CAD build for the part. Positions are in the model's coordinates, mm. A direction names the side the tool comes from. Coordinates: 2 decimals unless noted, no trailing zeros. Loops run counter-clockwise (first coordinate to the right, second up) from the corner with the lowest first, then second, coordinate; pieces in that order, holes last. Notation, with made-up numbers: (-23, -15.75) -> (12, -15.75) arc R11 cw to (12, -10.75) -> close; hole circle Ø4 at (-36.75, 0.5). An arc over 180 degrees is marked (long way). Answer as a JSON object with one key per item and string values. Group by question number.
from build123d import *

# Parameters (mm, degrees)
F0_W      = 12
F0_H      = 38.1
F1_DEPTH  = 50.8
F2_R      = 3.33175
F3_DEPTH  = 25.4
F4_W      = 25.4
F4_H      = 76.2
F4_W_2    = 38.1
F4_H_2    = 50.8
F4_W_3    = 12
F4_H_3    = 38.1
F4_H_4    = 25.4
F5_DEPTH  = 6.35
F7_DEPTH  = 1.905
F8_R      = 3.33175
F9_DEPTH  = 12.7
F10_R     = 5.08
F11_DEPTH = 15.24
F13_DEPTH = 2.54
F14_W     = 27.02
F14_H     = 33.02
F15_DEPTH = 6.351
F16_R     = 2.413
F17_DEPTH = 6.351


# Not quite as in the source:
# - a pattern or mirror of a feature is missing from the dataset's text; its kind, count and spacing are read off the source's solid


with BuildPart() as f1:
    # F0 (on Top) → F1 (new body)
    with BuildSketch(Plane.XY):
        Rectangle(F0_W, F0_H)
    extrude(amount=F1_DEPTH)

    # F2 (on face) → F3 (cut)
    with BuildSketch(Plane.XY.offset(50.8)):
        with Locations((0, 12.7)):
            Circle(F2_R)
        with Locations((0, -12.7)):
            Circle(F2_R)
    extrude(amount=-F3_DEPTH, mode=Mode.SUBTRACT)

    # F4 (on face) → F5 (join)
    with BuildSketch(Plane(origin=(0, 0, 0), x_dir=(1, 0, 0), z_dir=(0, 0, -1))):
        with Locations((0, 63.5)):
            Rectangle(F4_W, F4_H)
        with Locations((31.75, 0)):
            Rectangle(F4_W_2, F4_H_2)
        Rectangle(F4_W, F4_H_2)
        Rectangle(F4_W_3, F4_H_3, mode=Mode.SUBTRACT)
        with Locations((-31.75, 0)):
            Rectangle(F4_W_2, F4_H_2)
        with Locations((0, -38.1)):
            Rectangle(F4_W, F4_H_4)
    extrude(amount=-F5_DEPTH)

    # F6 (on Right) → F7 (join, symmetric)
    with BuildSketch(Plane.YZ):
        with BuildLine():
            Line((-19.05, 6.35), (-19.05, 22.86))
            add(Edge.make_bspline(
                [(-90.6148681487, 15.7624194539), (-19.05, 4.6606890297), (-19.05, 22.86)],
                knots=[4.0563179373, 4.0563179373, 4.0563179373, 6.2831853072, 6.2831853072, 6.2831853072], degree=2, weights=[1, 0.4415833544, 1]))
            ThreePointArc((-90.6148681487, 15.7624194539), (-98.2724942161, 13.5830277507), (-101.6, 6.35))
            Line((-101.6, 6.35), (-25.4, 6.35))
            Line((-25.4, 6.35), (-19.05, 6.35))
        make_face()
        with BuildLine():
            Line((19.05, 22.86), (19.05, 6.35))
            Line((19.05, 6.35), (25.4, 6.35))
            Line((25.4, 6.35), (50.8, 6.35))
            ThreePointArc((50.8, 6.35), (46.5346393393, 14.2911472106), (37.5586731715, 15.1200934946))
            add(Edge.make_bspline(
                [(19.05, 22.86), (19.05, 7.2770438497), (37.5586731715, 15.1200934946)],
                knots=[0, 0, 0, 2.0982208016, 2.0982208016, 2.0982208016], degree=2, weights=[1, 0.4983425099, 1]))
        make_face()
    extrude(amount=F7_DEPTH, both=True)

    # F8 (on face) → F9 (cut)
    with BuildSketch(Plane.XZ.offset(101.6)):
        with Locations((-7.62, 6.35)):
            Circle(F8_R)
        with Locations((7.62, 6.35)):
            Circle(F8_R)
    extrude(amount=-F9_DEPTH, mode=Mode.SUBTRACT)

    # F10 (on face) → F11 (join)
    with BuildSketch(Plane.XZ.offset(101.6)):
        with Locations((-7.62, 6.35)):
            Circle(F10_R)
        with BuildLine():
            ThreePointArc((-4.28825, 6.35), (-7.62, 3.01825), (-10.95175, 6.35))
            ThreePointArc((-10.95175, 6.35), (-7.62, 9.68175), (-4.28825, 6.35))
        make_face(mode=Mode.SUBTRACT)
        with Locations((7.62, 6.35)):
            Circle(F10_R)
        with BuildLine():
            ThreePointArc((10.95175, 6.35), (7.62, 3.01825), (4.28825, 6.35))
            ThreePointArc((4.28825, 6.35), (7.62, 9.68175), (10.95175, 6.35))
        make_face(mode=Mode.SUBTRACT)
    extrude(amount=-F11_DEPTH)

    # F12 (on face) → F13 (join)
    with BuildSketch(Plane(origin=(0, -86.36, 0), x_dir=(-1, 0, 0), z_dir=(0, 1, 0))):
        with BuildLine():
            ThreePointArc((-4.28825, 6.35), (-7.62, 9.68175), (-10.95175, 6.35))
            Line((-10.95175, 6.35), (-4.28825, 6.35))
        make_face()
        with BuildLine():
            ThreePointArc((10.95175, 6.35), (7.62, 9.68175), (4.28825, 6.35))
            Line((4.28825, 6.35), (10.95175, 6.35))
        make_face()
    extrude(amount=-F13_DEPTH)

    # F14 (on face) → F15 (cut, through all)
    with BuildSketch(Plane.XY.offset(6.35)):
        with Locations((-27.13, 0)):
            Rectangle(F14_W, F14_H)
        with Locations((28.4, 0)):
            Rectangle(F14_W, F14_H)
    extrude(amount=-F15_DEPTH, mode=Mode.SUBTRACT)

    # F16 (on face) → F17 (cut, through all)
    with BuildSketch(Plane.XY.offset(6.35)):
        with Locations((-7.3025, -73.66)):
            Circle(F16_R)
        with Locations((-7.3025, -38.1)):
            Circle(F16_R)
        with Locations((-45.72, -20.955)):
            Circle(F16_R)
        with Locations((-45.72, 20.955)):
            Circle(F16_R)
        with Locations((-7.3025, 38.1)):
            Circle(F16_R)
    f17 = extrude(amount=-F17_DEPTH, mode=Mode.SUBTRACT)

    # F17_copies: F17 across plane
    add(f17.mirror(Plane(origin=(0, 0, 0), x_dir=(0, 0, 1), z_dir=(1, 0, 0))), mode=Mode.SUBTRACT)


solid = f1.part
Item 1: Pull direction Z, two halves, no side cores. Call faces 1 (the cylindrical face through (-0.03, -98.18, 13.66)), 2 (the cylindrical face through (8.342, -95.339, 9.603)), 3 (the flat face through (-27, -16.51, 3)): +Z half, -Z half, draft (parallel to the pull), parting line (faces both ways), or undercut.
Item 2: Drill centre lines: L1, parallel to Y at x = 0, z = 46.5; L2, parallel to X at y = -38, z = 2; L3, parallel to X at y = -73, z = 3. Where is each one in solid material? Low to high.
Item 3: Band-saw the part on A-A, the plane x = 45.72. List the corners of the cut face in (y, z).
Item 4: 3-axis set-ups, long thin cutter, end or side, ignore diameter. For faces 4 (the flat face through (-32, 25.4, 3)), 5 (the flat face through (0, 19.05, 28)), 6 (the flat face through (1.905, 35, 11)), 7 (the flat face through (12.7, 38, 3)): which of +Z, -Z, +X, -X, +Y, -Y reach the whole face in a straight line?
Item 5: Band-saw the part on B-B, the plane y = -12.7. List the corners of the cut face in (x, z), and give its area (3 significant figures).
Item 6: Flat gauge pins, fed straight in: P1, Ø2.5, axis at x = -9.5, z = 9.5, coming from the +Y side; P2, Ø7.5, axis at x = 7.3, y = -38.1, coming from the +Z side; P3, Ø3, axis at x = -30, z = 2, coming from the +Y side; P4, Ø10.5, axis at x = 7.62, z = 6.35, coming from the -Y side. Where does each tip first touch, or does it go through?
Item 7: Band-saw the part on C-C, the plane x = -22. List the corners of the cut face in (y, z).
Item 8: Band-saw the part on D-D, the plane z = 29. List the corners of the cut face in (x, y), and give its area (3 significant figures).
Reply:
{
 "1": {"face 1": "+Z half", "face 2": "undercut", "face 3": "draft"},
 "2": {"L1": "-19.05 to -16.03, -9.37 to 9.37, 16.03 to 19.05", "L2": "-12.7 to -9.71, -4.89 to 4.89, 9.71 to 12.7", "L3": "-12.7 to -9.62, -4.98 to 4.98, 9.62 to 12.7"},
 "3": {"outline": "(-25.4, 0) -> (-23.37, 0) -> (-23.37, 6.35) -> (-25.4, 6.35) -> close; (-18.54, 0) -> (18.54, 0) -> (18.54, 6.35) -> (-18.54, 6.35) -> close; (23.37, 0) -> (25.4, 0) -> (25.4, 6.35) -> (23.37, 6.35) -> close"},
 "4": {"face 4": "+Z, -Z, -X, +Y", "face 5": "+Z, +Y", "face 6": "+Z, +X, +Y", "face 7": "+Z, -Z, +X, +Y"},
 "5": {"outline": "(-50.8, 0) -> (-40.64, 0) -> (-40.64, 6.35) -> (-50.8, 6.35) -> close; (-13.62, 0) -> (14.89, 0) -> (14.89, 6.35) -> (6, 6.35) -> (6, 50.8) -> (3.33, 50.8) -> (3.33, 25.4) -> (-3.33, 25.4) -> (-3.33, 50.8) -> (-6, 50.8) -> (-6, 6.35) -> (-13.62, 6.35) -> close; (41.91, 0) -> (50.8, 0) -> (50.8, 6.35) -> (41.91, 6.35) -> close", "area": "666 mm²"},
 "6": {"P1": "y = -86.36", "P2": "z = 6.35", "P3": "y = 25.4", "P4": "y = -101.6"},
 "7": {"outline": "(-25.4, 0) -> (-16.51, 0) -> (-16.51, 6.35) -> (-25.4, 6.35) -> close; (16.51, 0) -> (25.4, 0) -> (25.4, 6.35) -> (16.51, 6.35) -> close"},
 "8": {"outline": "(-6, -19.05) -> (6, -19.05) -> (6, 19.05) -> (-6, 19.05) -> close; hole circle Ø6.66 at (0, -12.7); hole circle Ø6.66 at (0, 12.7)", "area": "387 mm²"}
}
